```python
from build123d import *

# Parameters (mm, degrees)
SKETCH_1_R          = 3
EXTRUDE_1_DEPTH     = 2
FILLET_1_R          = 1
SKETCH_2_R          = 1.515
CUT_EXTRUDE_1_DEPTH = 10
CUT_EXTRUDE_2_DEPTH = 10
FILLET_2_R          = 1.3
SKETCH_4_W          = 31
SKETCH_4_H          = 10
CUT_EXTRUDE_3_DEPTH = 10
SKETCH_5_W          = 4
SKETCH_5_H          = 10
EXTRUDE_1_2_DEPTH   = 2
FILLET_4_R          = 1.5


with BuildPart() as part:
    # 草图1 → Extrude 1 (new body)
    with BuildSketch(Plane.XY):
        with BuildLine():
            Line((-20, -40), (20, -40))
            Line((20, -40), (20, -19))
            Line((20, -19), (11.781235871, 4.177616707))
            ThreePointArc((11.781235871, 4.177616707), (0, 12.5), (-11.781235871, 4.177616707))
            Line((-11.781235871, 4.177616707), (-20, -19))
            Line((-20, -19), (-20, -40))
        make_face()
        Circle(SKETCH_1_R, mode=Mode.SUBTRACT)
    extrude(amount=EXTRUDE_1_DEPTH)

    # 圆角1
    fillet_1_edges = [part.edges().sort_by_distance(p)[0] for p in [
        (20, -19, 1),
        (20, -40, 1),
        (-20, -40, 1),
        (-20, -19, 1),
    ]]
    fillet(fillet_1_edges, radius=FILLET_1_R)

    # 草图2 → 切除-拉伸1 (cut)
    with BuildSketch(Plane(origin=(0, 0, 0), x_dir=(-1, 0, 0), z_dir=(0, 0, -1))):
        with Locations((15, -37)):
            Circle(SKETCH_2_R)
        with Locations((-5, -37)):
            Circle(SKETCH_2_R)
    extrude(amount=-CUT_EXTRUDE_1_DEPTH, mode=Mode.SUBTRACT)

    # 草图3 → 切除-拉伸2 (cut)
    with BuildSketch(Plane(origin=(0, 0, 0), x_dir=(-1, 0, 0), z_dir=(0, 0, -1))):
        with BuildLine():
            Line((-7.539990958, 2.673674692), (-15.225458465, -19))
            Line((-15.225458465, -19), (15.225458465, -19))
            Line((15.225458465, -19), (7.539990958, 2.673674692))
            ThreePointArc((7.539990958, 2.673674692), (0, -8), (-7.539990958, 2.673674692))
        make_face()
    extrude(amount=-CUT_EXTRUDE_2_DEPTH, mode=Mode.SUBTRACT)

    # 圆角2
    fillet_2_edges = [part.edges().sort_by_distance(p)[0] for p in [
        (7.539990958, 2.673674692, 1),
        (-7.539990958, 2.673674692, 1),
        (-15.225458465, -19, 1),
        (15.225458465, -19, 1),
    ]]
    fillet(fillet_2_edges, radius=FILLET_2_R)

    # 草图4 → 切除-拉伸3 (cut)
    with BuildSketch(Plane(origin=(0, 0, 0), x_dir=(-1, 0, 0), z_dir=(0, 0, -1))):
        with Locations((0, -28)):
            Rectangle(SKETCH_4_W, SKETCH_4_H)
    extrude(amount=-CUT_EXTRUDE_3_DEPTH, mode=Mode.SUBTRACT)

    # 草图5 → Extrude 1 2 (add)
    with BuildSketch(Plane(origin=(0, 0, 0), x_dir=(-1, 0, 0), z_dir=(0, 0, -1))):
        with Locations((0, -28)):
            Rectangle(SKETCH_5_W, SKETCH_5_H)
    extrude(amount=-EXTRUDE_1_2_DEPTH)

    # 圆角4
    fillet_4_edges = [part.edges().sort_by_distance(p)[0] for p in [
        (15.5, -33, 1),
        (15.5, -23, 1),
        (-15.5, -23, 1),
        (-15.5, -33, 1),
        (2, -33, 1),
        (2, -23, 1),
        (-2, -23, 1),
        (-2, -33, 1),
    ]]
    fillet(fillet_4_edges, radius=FILLET_4_R)


solid = part.part
```
Could you check a few things on this model? Use its own coordinates, in mm. A direction names the side the tool comes from. Give positions to 0.01 mm unless a question says otherwise; leave off trailing zeros. Order: outer loops, then holes, each group sorted by start corner. A loop starts at its lowest first (then second) coordinate and runs counter-clockwise, first axis right, second up.
Q1. If I drill on line 1 along Y through (x, z) = (0, 1.05); line 2 along Y through (x, z) = (2.5, 1.4); line 3 along X through (y, z) = (-6.5, 1), over which ranges is the centre line in solid material (lowest first)?
Q2. Suppose I cut it at A-A, the plane y = -37. Write out the boundary of the cut face in (x, z) (3 decimals).
Q3. Suppose I cut it at B-B, the plane x = 0. Write out the boundary of the cut face in (y, z), and give its area (3 significant figures).
Q4. Suppose I cut it at C-C, the plane y = 1. Write out the boundary of the cut face in (x, z).
Q5. Suppose I cut it at D-D, the plane x = 5. Write out the boundary of the cut face in (y, z) (3 decimals), and give its area (3 significant figures).
Q6. I'm going to push flat-ended pins straight in: P1, Ø1, axis at x = -6, z = 1, coming from the +Y side (3 decimals); P2, Ø2.5, axis at x = -15, y = -37, coming from the -Z side. Where does each tip first touch, or does it pass through?
Q7. We'd pull the mould along X, two halves only. Please class faces 3 (the flat face through (-0.3, -19.2, 0)), 4 (the flat face through (0, -19, 1)), 5 (the cylindrical face through (-19.699, -39.715, 1.014)), 6 (the cylindrical face through (-15.07, -32.55, 1.01)): +X half, -X half, draft (parallel to the pull), parting line (faces both ways), or undercut.
Q8. For faces 1 (the cylindrical face through (8.5, -2.54, 1.01)), 2 (the flat face through (0, -40, 1)), which set-ups out of +Z, -Z, +X, -X, +Y, -Y let a thin tool reach every point of the face, with its end or its side?
Solution:
1. line 1: y = -40 to -19, -8 to -3, 3 to 12.5
1. line 2: y = -40 to -32.62, -23.38 to -19, -7.6 to -1.66, 1.66 to 12.25
1. line 3: x = -15.57 to -10.79, -4.66 to 4.66, 10.79 to 15.57
2. outline: (-20, 0) - (-16.515, 0) - (-16.515, 2) - (-20, 2) - close; (-13.485, 0) - (3.485, 0) - (3.485, 2) - (-13.485, 2) - close; (6.515, 0) - (20, 0) - (20, 2) - (6.515, 2) - close
3. outline: (-40, 0) - (-19, 0) - (-19, 2) - (-40, 2) - close; (-8, 0) - (-3, 0) - (-3, 2) - (-8, 2) - close; (3, 0) - (12.5, 0) - (12.5, 2) - (3, 2) - close
3. area: 71.0 mm2
4. outline: (-12.91, 0) - (-2.83, 0) - (-2.83, 2) - (-12.91, 2) - close; (2.83, 0) - (12.91, 0) - (12.91, 2) - (2.83, 2) - close
5. outline: (-40, 0) - (-38.515, 0) - (-38.515, 2) - (-40, 2) - close; (-35.485, 0) - (-33, 0) - (-33, 2) - (-35.485, 2) - close; (-23, 0) - (-19, 0) - (-19, 2) - (-23, 2) - close; (-6.245, 0) - (11.456, 0) - (11.456, 2) - (-6.245, 2) - close
5. area: 51.3 mm2
6. P1: stops at y = 11.225
6. P2: passes through
7. face 3: draft
7. face 4: undercut
7. face 5: -X half
7. face 6: undercut
8. face 1: +Z, -Z
8. face 2: +Z, -Z, +X, -X, -Y
